Geometry check sheet. Reference: the model listing, model coordinates, mm. A direction names the side the tool comes from. Give positions to 0.01 mm unless a question says otherwise; leave off trailing zeros. Write each loop counter-clockwise with the first axis right and the second up, starting at its lowest first coordinate (ties: lowest second). Pieces come first, ordered by that corner, then holes. Notation, with made-up numbers: (40.5, -31.5) - (51.5, -31.5) arc R30 cw to (51.5, -3.5) - close; hole circle Ø2 at (72.25, 33.25). An arc over 180 degrees is marked (long way). One line per question, with ' | ' between items. Start each with the question number.
Q1. Section check C-C on z = 8.5. Record the boundary of the cut face in (x, y).
Q2. Set-up check for faces 1 (the face through (-0.65, 13.7, 7.31)), 2 (the face through (-35, 0, 5)): record each of +Z, -Z, +X, -X, +Y, -Y from which the full face is reachable in a straight line by a thin tool's end or side.
Q3. Release check for a two-part mould opening along Y. For faces 3 (the face through (0, 0, 0)), 4 (the face through (0, -25, 5)), 5 (the face through (0.325, 6.264, 2.477)) record: +Y half, -Y half, draft (parallel to the pull), parting line (faces both ways), or undercut.
Q4. Section check A-A on x = 0. Record the boundary of the cut face in (y, z) (3 decimals), and give its area (3 significant figures).
Q5. Section check B-B on y = 12.5. Record the boundary of the cut face in (x, z) (3 decimals), and give its area (3 significant figures).
Q6. Thickness scan on L1, parallel to X at y = 8.5, z = 2.75; L2, parallel to Y at x = 0, z = 2.25; L3, parallel to Y at x = -2.5, z = 8.25. Record the ranges inside material, lowest first. Write a range as [from, to].
Q7. Gauge pin test, flat end, axial feed: P1, Ø3, axis at x = 0, y = 8.74, coming from the +Z side. Record the tip position at first contact, or that the pin passes through.
```python
from build123d import *

# Parameters (mm, degrees)
CROQUIS1_W              = 70
CROQUIS1_H              = 50
CROQUIS1_R              = 2.5
SALIENTE_EXTRUIR1_DEPTH = 9.525
CROQUIS2_R              = 5
CORTAR_EXTRUIR1_DEPTH   = 4.5


with BuildPart() as part:
    # Croquis1 → Saliente-Extruir1 (new body)
    with BuildSketch(Plane.XY):
        Rectangle(CROQUIS1_W, CROQUIS1_H)
        with Locations(Location((0, 8.742399315, 0), (0, 0, 180))):
            Circle(CROQUIS1_R, mode=Mode.SUBTRACT)
    extrude(amount=SALIENTE_EXTRUIR1_DEPTH)

    # Croquis2 → Cortar-Extruir1 (cut)
    with BuildSketch(Plane.XY.offset(9.525)):
        with Locations((0, 8.742399315)):
            Circle(CROQUIS2_R)
    extrude(amount=-CORTAR_EXTRUIR1_DEPTH, mode=Mode.SUBTRACT)


solid = part.part
```
Working result:
1) outline: (-35, -25) - (35, -25) - (35, 25) - (-35, 25) - close; hole circle Ø10 at (0, 8.74)
2) face 1: +Z | face 2: +Z, -Z, -X, +Y, -Y
3) face 3: draft | face 4: -Y half | face 5: undercut
4) outline: (-25, 0) - (6.242, 0) - (6.242, 5.025) - (3.742, 5.025) - (3.742, 9.525) - (-25, 9.525) - close; (11.242, 0) - (25, 0) - (25, 9.525) - (13.742, 9.525) - (13.742, 5.025) - (11.242, 5.025) - close | area: 406 mm2
5) outline: (-35, 0) - (35, 0) - (35, 9.525) - (3.299, 9.525) - (3.299, 5.025) - (-3.299, 5.025) - (-3.299, 9.525) - (-35, 9.525) - close | area: 637 mm2
6) L1: x = [-35, -2.49], [2.49, 35] | L2: y = [-25, 6.24], [11.24, 25] | L3: y = [-25, 4.41], [13.07, 25]
7) P1: passes through
